Design review of the part built by this model. Coordinates are the model's own, in mm. Round coordinates to 2 decimals unless told otherwise and drop trailing zeros. Use a Markdown table: item, result.
from build123d import *

# Parameters (mm, degrees)
SKICA1_R                 = 0.5
SKICA1_R_2               = 2.3
SKICA1_R_3               = 0.9
SKICA1_W                 = 3
SKICA1_H                 = 13
SKICA1_H_2               = 5.5
SKICA1_W_2               = 17.6
SKICA1_H_3               = 10.6
SKICA1_W_3               = 12.4
SKICA1_H_4               = 24
SKICA1_W_4               = 2.8
SKICA1_W_5               = 3.2
SKICA1_H_5               = 10
SKICA1_W_6               = 4.6
SKICA1_H_6               = 4.6
P_IDAT_VYSUNUT_M1_DEPTH  = 3
SKICA2_R                 = 1.5
ODEBRAT_VYSUNUT_M1_DEPTH = 3
ZKOSEN_1_SIZE            = 1.5
ZAOBLIT1_R               = 40
ZAOBLIT2_R               = 4
SKICA3_R                 = 0.5
SKICA3_W                 = 2.8
SKICA3_H                 = 13
ODEBRAT_VYSUNUT_M2_DEPTH = 129.730338305
SKICA7_R                 = 4
ODEBRAT_VYSUNUT_M3_DEPTH = 129.730338305


with BuildPart() as part:
    # Skica1 → Přidat vysunutím1 (new body)
    with BuildSketch(Plane.XY):
        Polygon((-62.5, -32.5), (-62.5, 32.5), (-32.5, 62.5), (-19.003438856, 112.5), (19.003438856, 112.5), (32.5, 62.5), (62.5, 32.5), (62.5, -32.5), (32.5, -62.5), (-32.5, -62.5), align=None)
        with Locations((0, 100.5)):
            Circle(SKICA1_R, mode=Mode.SUBTRACT)
        with Locations(Location((0, 72.5, 0), (0, 0, 180))):
            Circle(SKICA1_R, mode=Mode.SUBTRACT)
        with Locations((0, 108.5)):
            Circle(SKICA1_R_2, mode=Mode.SUBTRACT)
        with Locations((7.97, 108.5)):
            Circle(SKICA1_R_2, mode=Mode.SUBTRACT)
        with Locations((15.94, 108.5)):
            Circle(SKICA1_R_2, mode=Mode.SUBTRACT)
        with Locations(Location((-15.94, 108.5, 0), (0, 0, 180))):
            Circle(SKICA1_R_2, mode=Mode.SUBTRACT)
        with Locations(Location((-7.97, 108.5, 0), (0, 0, 180))):
            Circle(SKICA1_R_2, mode=Mode.SUBTRACT)
        with Locations(Location((-18.017013584, 100.805397049, 0), (0, 0, 180))):
            Circle(SKICA1_R_2, mode=Mode.SUBTRACT)
        with Locations((-20.094027168, 93.110794098)):
            Circle(SKICA1_R_2, mode=Mode.SUBTRACT)
        with Locations((-22.171040752, 85.416191147)):
            Circle(SKICA1_R_2, mode=Mode.SUBTRACT)
        with Locations((-24.248054336, 77.721588196)):
            Circle(SKICA1_R_2, mode=Mode.SUBTRACT)
        with Locations(Location((24.248054336, 77.721588196, 0), (0, 0, 180))):
            Circle(SKICA1_R_2, mode=Mode.SUBTRACT)
        with Locations(Location((22.171040752, 85.416191147, 0), (0, 0, 180))):
            Circle(SKICA1_R_2, mode=Mode.SUBTRACT)
        with Locations(Location((20.094027168, 93.110794098, 0), (0, 0, 180))):
            Circle(SKICA1_R_2, mode=Mode.SUBTRACT)
        with Locations((18.017013584, 100.805397049)):
            Circle(SKICA1_R_2, mode=Mode.SUBTRACT)
        with Locations((47.397781356, 0)):
            Circle(SKICA1_R_3, mode=Mode.SUBTRACT)
        with Locations(Location((26.897781356, 0, 0), (0, 0, 180))):
            Circle(SKICA1_R_3, mode=Mode.SUBTRACT)
        with Locations(Location((-47.397781356, 0, 0), (0, 0, 180))):
            Circle(SKICA1_R_3, mode=Mode.SUBTRACT)
        with Locations((-26.897781356, 0)):
            Circle(SKICA1_R_3, mode=Mode.SUBTRACT)
        Polygon((-44.147781356, 3.2), (-38.647781356, 3.2), (-38.647781356, 7.5), (-35.647781356, 7.5), (-35.647781356, 3.2), (-30.147781356, 3.2), (-30.147781356, -3.2), (-35.647781356, -3.2), (-35.647781356, -7.5), (-38.647781356, -7.5), (-38.647781356, -3.2), (-44.147781356, -3.2), align=None, mode=Mode.SUBTRACT)
        with Locations((-43.047781356, 20.7)):
            Rectangle(SKICA1_W, SKICA1_H, mode=Mode.SUBTRACT)
        with Locations((-52.847781356, 0)):
            Rectangle(SKICA1_W, SKICA1_H_2, mode=Mode.SUBTRACT)
        with Locations((-43.047781356, -20.7)):
            Rectangle(SKICA1_W, SKICA1_H, mode=Mode.SUBTRACT)
        Polygon((38.647781356, -7.5), (35.647781356, -7.5), (35.647781356, -3.2), (30.147781356, -3.2), (30.147781356, 3.2), (35.647781356, 3.2), (35.647781356, 7.5), (38.647781356, 7.5), (38.647781356, 3.2), (44.147781356, 3.2), (44.147781356, -3.2), (38.647781356, -3.2), align=None, mode=Mode.SUBTRACT)
        with Locations((52.847781356, 0)):
            Rectangle(SKICA1_W, SKICA1_H_2, mode=Mode.SUBTRACT)
        with Locations((43.047781356, 20.7)):
            Rectangle(SKICA1_W, SKICA1_H, mode=Mode.SUBTRACT)
        with Locations((43.047781356, -20.7)):
            Rectangle(SKICA1_W, SKICA1_H, mode=Mode.SUBTRACT)
        with Locations((16.7, 53.8)):
            Rectangle(SKICA1_W_2, SKICA1_H_3, mode=Mode.SUBTRACT)
        with Locations((-16.7, 53.8)):
            Rectangle(SKICA1_W_2, SKICA1_H_3, mode=Mode.SUBTRACT)
        with Locations((0, 86.5)):
            Rectangle(SKICA1_W_3, SKICA1_H_4, mode=Mode.SUBTRACT)
        with Locations((-12.4, 86.5)):
            Rectangle(SKICA1_W_4, SKICA1_H, mode=Mode.SUBTRACT)
        Polygon((-20.487479207, 65.088190451), (-10.828220944, 62.5), (-10, 65.590962644), (-19.659258263, 68.179153095), align=None, mode=Mode.SUBTRACT)
        with Locations((12.4, 86.5)):
            Rectangle(SKICA1_W_4, SKICA1_H, mode=Mode.SUBTRACT)
        with Locations((31.6, 31)):
            Rectangle(SKICA1_W_5, SKICA1_H_5, mode=Mode.SUBTRACT)
        with Locations((-31.6, 31)):
            Rectangle(SKICA1_W_5, SKICA1_H_5, mode=Mode.SUBTRACT)
        with Locations((25.3, 20.23)):
            Rectangle(SKICA1_W_6, SKICA1_H_6, mode=Mode.SUBTRACT)
        with Locations((25.3, -51.5)):
            Rectangle(SKICA1_W_6, SKICA1_H_6, mode=Mode.SUBTRACT)
        with Locations((-25.3, -51.5)):
            Rectangle(SKICA1_W_6, SKICA1_H_6, mode=Mode.SUBTRACT)
        with Locations((-25.3, 20.23)):
            Rectangle(SKICA1_W_6, SKICA1_H_6, mode=Mode.SUBTRACT)
    extrude(amount=P_IDAT_VYSUNUT_M1_DEPTH)

    # Skica2 → Odebrat vysunutím1 (cut)
    with BuildSketch(Plane.XY):
        with Locations(Location((0, 39.6, 0), (0, 0, 180))):
            Circle(SKICA2_R)
        with Locations(Location((0, 55.6, 0), (0, 0, 180))):
            Circle(SKICA2_R)
        with Locations(Location((0, -55.6, 0), (0, 0, 180))):
            Circle(SKICA2_R)
        with Locations(Location((0, -39.6, 0), (0, 0, 180))):
            Circle(SKICA2_R)
    extrude(amount=ODEBRAT_VYSUNUT_M1_DEPTH, mode=Mode.SUBTRACT)

    # Zkosení1
    zkosen_1_edges = [part.edges().sort_by_distance(p)[0] for p in [
        (1.5, 55.6, 3),
        (1.5, -55.6, 3),
        (1.5, -39.6, 3),
        (1.5, 39.6, 3),
    ]]
    chamfer(zkosen_1_edges, length=ZKOSEN_1_SIZE)

    # Zaoblit1
    zaoblit1_edges = [part.edges().sort_by_distance(p)[0] for p in [
        (-62.5, -32.5, 1.5),
        (-62.5, 32.5, 1.5),
        (-32.5, 62.5, 1.5),
        (32.5, 62.5, 1.5),
        (62.5, 32.5, 1.5),
        (62.5, -32.5, 1.5),
        (32.5, -62.5, 1.5),
        (-32.5, -62.5, 1.5),
    ]]
    fillet(zaoblit1_edges, radius=ZAOBLIT1_R)

    # Zaoblit2
    zaoblit2_edges = [part.edges().sort_by_distance(p)[0] for p in [
        (-19.003438856, 112.5, 1.5),
        (19.003438856, 112.5, 1.5),
    ]]
    fillet(zaoblit2_edges, radius=ZAOBLIT2_R)

    # Skica3 → Odebrat vysunutím2 (cut, through all)
    with BuildSketch(Plane.XY.offset(3)):
        with Locations((-28.2, 41.3)):
            Circle(SKICA3_R)
        with Locations(Location((28.2, 41.3, 0), (0, 0, 180))):
            Circle(SKICA3_R)
        with Locations((0, -50.6)):
            Rectangle(SKICA3_W, SKICA3_H)
    extrude(amount=-ODEBRAT_VYSUNUT_M2_DEPTH, mode=Mode.SUBTRACT)

    # Skica7 → Odebrat vysunutím3 (cut, through all)
    with BuildSketch(Plane.XY.offset(3)):
        with Locations((-38.5, -39.5)):
            Circle(SKICA7_R)
        with Locations((38.5, -39.5)):
            Circle(SKICA7_R)
        with Locations((-37.5, 44)):
            Circle(SKICA7_R)
        with Locations((37.5, 44)):
            Circle(SKICA7_R)
    extrude(amount=-ODEBRAT_VYSUNUT_M3_DEPTH, mode=Mode.SUBTRACT)


solid = part.part
1. Take a section at A-A on z = 0.8. Count the separate pieces of the cut face and the enclosed holes in it, and give its area (3 significant figures).
Check values:
| item | result |
|---|---|
| separate pieces | 1 |
| enclosed holes | 49 |
| area | 14,400 mm² |
2. Insertion check: pin 1 (1.5 mm diameter, centred on x = -52.5, z = 1, fed in from -Y); pin 2 (0.9 mm diameter, centred on x = 26, z = 2, fed in from -Y); pin 3 (1.5 mm diameter, centred on x = -41.5, z = 1, fed in from +Y); pin 4 (4 mm diameter, centred on x = 15.94, y = 108.5, fed in from +Z). Each pin has a flat end and moves straight along its axis. Give the tip position at first contact, or say it passes through.
Check values:
| item | result |
|---|---|
| pin 1 | stops at y = -43.22 |
| pin 2 | stops at y = -61.33 |
| pin 3 | stops at y = 54.25 |
| pin 4 | passes through |
3. The part is to be moulded in two halves that separate along X. For faces 1 (the face through (-47, -48, 1)), 2 (the face through (22.47, 83.136, 1.479)), 3 (the face through (31.035, -59.539, 1.521)), 4 (the face through (1, 7, 3)), say which applies: pulls with the +X half, pulls with the -X half, needs draft (parallel to the pull), parting line crosses it, or undercut.
Check values:
| item | result |
|---|---|
| face 1 | pulls with the -X half |
| face 2 | undercut |
| face 3 | pulls with the +X half |
| face 4 | needs draft |
4. Wall thickness on line 1 along Y through (x, z) = (15.94, 0.9); line 2 along X through (y, z) = (88, 0.2); line 3 along X through (y, z) = (-38, 2.75): over which ranges is each line inside the solid? List them lowest first. Write a range as from..to.
Check values:
| item | result |
|---|---|
| line 1 | y = -62.5..48.5, 59.1..99.82, 101.79..106.2, 110.8..112.5 |
| line 2 | x = -25.62..-13.8, -11..-6.2, 6.2..11, 13.8..25.62 |
| line 3 | x = -55.86..-42.21, -34.79..-2.24, 2.24..34.79, 42.21..55.86 |
